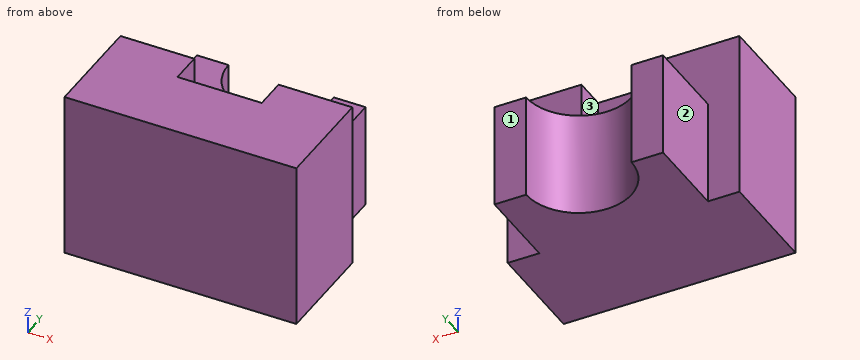
```python
from build123d import *

# Parameters (mm, degrees)
SKETCH3_W               = 110
SKETCH3_H               = 80
BOSS_EXTRUDE2_DEPTH     = 50
SKETCH6_W               = 80
SKETCH6_H               = 50
BOSS_EXTRUDE3_DEPTH     = 90
SKETCH7_R               = 25
CUT_EXTRUDE1_DEPTH      = 133.382022949
CUT_EXTRUDE2_DEPTH      = 133.382022949
CUT_EXTRUDE2_DEPTH_BACK = 30
SKETCH8_W               = 40
SKETCH8_H               = 15


with BuildPart() as part:
    # Sketch3 → Boss-Extrude2 (new body)
    with BuildSketch(Plane(origin=(0, 0, 0), x_dir=(1, 0, 0), z_dir=(0, 1, 0))):
        Rectangle(SKETCH3_W, SKETCH3_H)
    extrude(amount=BOSS_EXTRUDE2_DEPTH)

    # Sketch6 → Boss-Extrude3 (add)
    with BuildSketch(Plane.XZ):
        with Locations((0, -15)):
            Rectangle(SKETCH6_W, SKETCH6_H)
    extrude(amount=-BOSS_EXTRUDE3_DEPTH)

    # Sketch7 → Cut-Extrude1 (cut, through all)
    with BuildSketch(Plane(origin=(0, 0, -40), x_dir=(-1, 0, 0), z_dir=(0, 0, -1))):
        with Locations((0, 90)):
            Circle(SKETCH7_R)
    extrude(amount=-CUT_EXTRUDE1_DEPTH, mode=Mode.SUBTRACT)

    # Sketch8 → Cut-Extrude2 (cut, two sides: drawn at the far end of the back side and taken through both)
    with BuildSketch(Plane.XY.offset(40).offset(-CUT_EXTRUDE2_DEPTH_BACK)):
        with Locations((0, 42.5)):
            Rectangle(SKETCH8_W, SKETCH8_H)
    extrude(amount=CUT_EXTRUDE2_DEPTH + CUT_EXTRUDE2_DEPTH_BACK, mode=Mode.SUBTRACT)


solid = part.part
```
Verification items for the finished model (mm, model axes). Face numbers are marked on the shaded views. Coordinates: 2 decimals unless noted, no trailing zeros. Loops run counter-clockwise (first coordinate to the right, second up) from the corner with the lowest first, then second, coordinate; pieces in that order, holes last. Notation, with made-up numbers: (3.25, 18.5) -> (56.25, 18.5) arc R22 ccw to (56.25, 34.5) -> close; hole circle Ø6 at (40.5, 5). An arc over 180 degrees is marked (long way). Answer in a Markdown table with one row per item.
1) Draft check along X on the marked faces 1, 2 and 3. Enter one of: released by +X, released by -X, zero draft, split by the parting line, or undercut.
The answers:
| item | result |
|---|---|
| face 1 | zero draft |
| face 2 | released by -X |
| face 3 | undercut |
2) Section check C-C (y = 47). Record the cut outline in (x, z).
The answers:
| item | result |
|---|---|
| outline | (-55, -40) -> (55, -40) -> (55, 40) -> (20, 40) -> (20, 10) -> (-20, 10) -> (-20, 40) -> (-55, 40) -> close |
3) Depth check by flat-ended pin: P1, Ø20, axis at y = 75, z = -6, coming from the -X side; P2, Ø3, axis at x = 18.5, y = 72, coming from the +Z side. Enter the tip coordinate at first touch or a pass-through.
The answers:
| item | result |
|---|---|
| P1 | stops at x = -40 |
| P2 | stops at z = 10 |
4) Section check D-D (z = 27). Record the cut outline in (x, y), and give its area (3 significant figures).
The answers:
| item | result |
|---|---|
| outline | (-55, 0) -> (55, 0) -> (55, 50) -> (20, 50) -> (20, 35) -> (-20, 35) -> (-20, 50) -> (-55, 50) -> close |
| area | 4,900 mm2 |
5) Scan lines: line 1 along Y through (x, z) = (-20.5, 12.5); line 2 along X through (y, z) = (46, 25.5); line 3 along Y through (x, z) = (-18, 24). Record each from-to range of solid material in increasing order. Write a range as from..to.
The answers:
| item | result |
|---|---|
| line 1 | y = 0..50 |
| line 2 | x = -55..-20, 20..55 |
| line 3 | y = 0..35 |
6) Section check A-A (y = 71.5). Record the cut outline in (x, z).
The answers:
| item | result |
|---|---|
| outline | (-40, -40) -> (-16.82, -40) -> (-16.82, 10) -> (-40, 10) -> close; (16.82, -40) -> (40, -40) -> (40, 10) -> (16.82, 10) -> close |
7) Section check B-B (x = 0). Record the cut outline in (y, z).
The answers:
| item | result |
|---|---|
| outline | (0, -40) -> (65, -40) -> (65, 10) -> (35, 10) -> (35, 40) -> (0, 40) -> close |
